Verification items for the finished model (mm, model axes). Face numbers are marked on the shaded views. A direction names the side the tool comes from. Coordinates: 2 decimals unless noted, no trailing zeros. Order: outer loops, then holes, each group sorted by start corner. A loop starts at its lowest first (then second) coordinate and runs counter-clockwise, first axis right, second up. Notation, with made-up numbers: (-21.75, 21.5) - (-6.75, 21.5) arc R33 cw to (-6.75, 54.5) - close; hole circle Ø2 at (45, -17). An arc over 180 degrees is marked (long way). One line per question, with ' | ' between items. Start each with the question number.
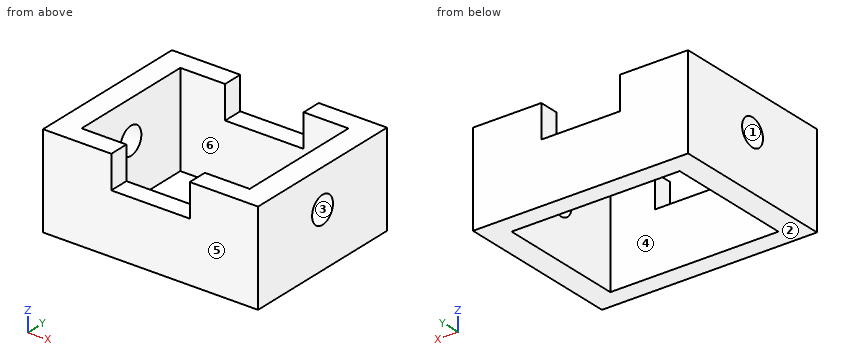
from build123d import *

# Parameters (mm, degrees)
F0_W     = 151.84383
F0_H     = 118.781612
F0_W_2   = 118.697516
F0_H_2   = 90.967916
F1_DEPTH = 50.8
F2_DEPTH = 65.532
F3_W     = 55.418182
F3_H     = 23.22946
F4_DEPTH = 118.782611
F5_R     = 9.604265
F6_DEPTH = 151.844831


with BuildPart() as f1:
    # F0 (on Top) → F1 (new body)
    with BuildSketch(Plane.XY):
        Rectangle(F0_W, F0_H)
        Rectangle(F0_W_2, F0_H_2, mode=Mode.SUBTRACT)
    extrude(amount=F1_DEPTH)

    # F0 (on Top) → F2 (join)
    with BuildSketch(Plane.XY):
        Rectangle(F0_W, F0_H)
        Rectangle(F0_W_2, F0_H_2, mode=Mode.SUBTRACT)
    extrude(amount=F2_DEPTH)

    # F3 (on face) → F4 (cut, through all)
    with BuildSketch(Plane.XZ.offset(59.390806)):
        with Locations((0, 53.91727)):
            Rectangle(F3_W, F3_H)
    extrude(amount=-F4_DEPTH, mode=Mode.SUBTRACT)

    # F5 (on face) → F6 (cut, through all)
    with BuildSketch(Plane.YZ.offset(75.921915)):
        with Locations((0, 38.446363)):
            Circle(F5_R)
    extrude(amount=-F6_DEPTH, mode=Mode.SUBTRACT)


solid = f1.part
Item 1: Gauge pin test, flat ends, axial feed: pin 1 (7 mm diameter, centred on x = -0.5, y = -52.5, fed in from +Z); pin 2 (5 mm diameter, centred on x = 24.5, z = 58.5, fed in from -Y). Record the tip position at first contact, or that the pin passes through.
Item 2: Section check D-D (z = 10.5). Record the cut outline in (x, y).
Item 3: Thickness scan on probe 1 along Y at (x, z) = (-3.5, 8); probe 2 along X at (y, z) = (35.5, 7.5); probe 3 along Z at (x, y) = (71, 0). Record the ranges inside material, lowest first. Write a range as from..to.
Item 4: Section check C-C (y = 14). Record the cut outline in (x, z).
Item 5: Set-up check for the marked faces 5 and 6: record each of +Z, -Z, +X, -X, +Y, -Y from which the full face is reachable in a straight line by a thin tool's end or side.
Item 6: Mould release check, pull along Z, two halves, no side actions. Record for the marked faces 1, 2, 3 and 4: +Z half, -Z half, draft (parallel to the pull), parting line (faces both ways), or undercut.
Item 7: Section check B-B (y = 0). Record the cut outline in (x, z), then the cut area to 3 significant figures.
Item 8: Section check A-A (z = 51.5). Record the cut outline in (x, y), then the cut area to 3 significant figures.
Completed:
1) pin 1: stops at z = 42.3 | pin 2: passes through
2) outline: (-75.92, -59.39) - (75.92, -59.39) - (75.92, 59.39) - (-75.92, 59.39) - close; hole (-59.35, -45.48) - (59.35, -45.48) - (59.35, 45.48) - (-59.35, 45.48) - close
3) probe 1: y = -59.39..-45.48, 45.48..59.39 | probe 2: x = -75.92..-59.35, 59.35..75.92 | probe 3: z = 0..28.84, 48.05..65.53
4) outline: (-75.92, 0) - (-59.35, 0) - (-59.35, 65.53) - (-75.92, 65.53) - close; (59.35, 0) - (75.92, 0) - (75.92, 65.53) - (59.35, 65.53) - close
5) face 5: +Z, -Z, +X, -X, -Y | face 6: +Z, -Z
6) face 1: undercut | face 2: -Z half | face 3: undercut | face 4: draft
7) outline: (-75.92, 0) - (-59.35, 0) - (-59.35, 28.84) - (-75.92, 28.84) - close; (-75.92, 48.05) - (-59.35, 48.05) - (-59.35, 65.53) - (-75.92, 65.53) - close; (59.35, 0) - (75.92, 0) - (75.92, 28.84) - (59.35, 28.84) - close; (59.35, 48.05) - (75.92, 48.05) - (75.92, 65.53) - (59.35, 65.53) - close | area: 1,540 mm^2
8) outline: (-75.92, -59.39) - (-27.71, -59.39) - (-27.71, -45.48) - (-59.35, -45.48) - (-59.35, 45.48) - (-27.71, 45.48) - (-27.71, 59.39) - (-75.92, 59.39) - close; (27.71, -59.39) - (75.92, -59.39) - (75.92, 59.39) - (27.71, 59.39) - (27.71, 45.48) - (59.35, 45.48) - (59.35, -45.48) - (27.71, -45.48) - close | area: 5,700 mm^2
